Can you work these out from the model? Positions are in its coordinate system, mm. Coordinates: 2 decimals unless noted, no trailing zeros. Write each loop counter-clockwise with the first axis right and the second up, starting at its lowest first coordinate (ties: lowest second). Pieces come first, ordered by that corner, then holes. Notation, with made-up numbers: (-6.5, -2.5) -> (48.5, -2.5) arc R24 ccw to (48.5, 26.5) -> close; hole circle Ø9 at (28, 56.5). An arc over 180 degrees is marked (long way). Use one line per item in the form item = value.
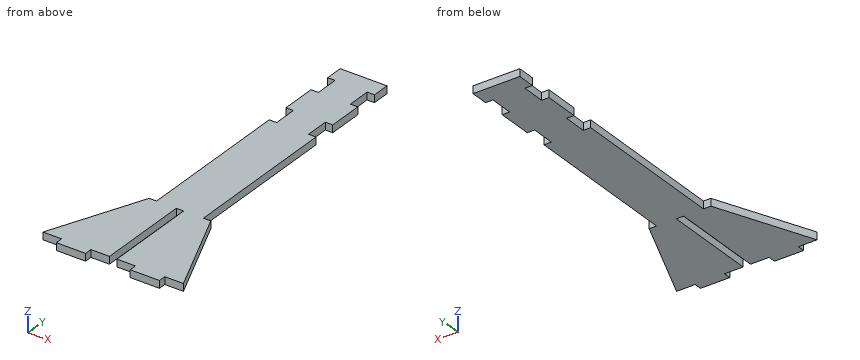
```python
from build123d import *

# Parameters (mm, degrees)
BOSS_EXTRU_1_DEPTH      = 6.35
ENL_V_MAT_EXTRU_1_REACH = 308.007
ESQUISSE2_W             = 6.35
ESQUISSE2_H             = 80
ENL_V_MAT_EXTRU_2_REACH = 308.007
ESQUISSE4_W             = 6.35
ESQUISSE4_H             = 20
SKETCH2_W               = 25
SKETCH2_H               = 6.35
BOSS_EXTRUDE2_DEPTH     = 6.35


with BuildPart() as part:
    # Esquisse1 → Boss.-Extru.1 (new body)
    with BuildSketch(Plane.XY):
        Polygon((-20, 300), (20, 300), (20, 80), (26.35, 80), (60, 0), (-60, 0), (-26.35, 80), (-20, 80), align=None)
    extrude(amount=BOSS_EXTRU_1_DEPTH)

    # Esquisse2 → Enlèv. mat.-Extru.1 (cut, up to next)
    with BuildSketch(Plane.XY.offset(6.35), mode=Mode.PRIVATE) as enl_v_mat_extru_1_sk1:
        with Locations((0, 40)):
            Rectangle(ESQUISSE2_W, ESQUISSE2_H)
    enl_v_mat_extru_1_tool1 = extrude(enl_v_mat_extru_1_sk1.sketch, amount=-ENL_V_MAT_EXTRU_1_REACH, mode=Mode.PRIVATE) & part.part
    add(enl_v_mat_extru_1_tool1.solids().sort_by_distance((0, 40, 6.35))[0], mode=Mode.SUBTRACT)

    # Esquisse4 → Enlèv. mat.-Extru.2 (cut, up to next)
    with BuildSketch(Plane.XY.offset(6.35), mode=Mode.PRIVATE) as enl_v_mat_extru_2_sk1:
        with Locations((16.825, 225)):
            Rectangle(ESQUISSE4_W, ESQUISSE4_H)
    enl_v_mat_extru_2_tool1 = extrude(enl_v_mat_extru_2_sk1.sketch, amount=-ENL_V_MAT_EXTRU_2_REACH, mode=Mode.PRIVATE) & part.part
    # Esquisse4 → Enlèv. mat.-Extru.2 (cut, up to next)
    with BuildSketch(Plane.XY.offset(6.35), mode=Mode.PRIVATE) as enl_v_mat_extru_2_sk2:
        with Locations((-16.825, 225)):
            Rectangle(ESQUISSE4_W, ESQUISSE4_H)
    enl_v_mat_extru_2_tool2 = extrude(enl_v_mat_extru_2_sk2.sketch, amount=-ENL_V_MAT_EXTRU_2_REACH, mode=Mode.PRIVATE) & part.part
    # Esquisse4 → Enlèv. mat.-Extru.2 (cut, up to next)
    with BuildSketch(Plane.XY.offset(6.35), mode=Mode.PRIVATE) as enl_v_mat_extru_2_sk3:
        with Locations((-16.825, 275)):
            Rectangle(ESQUISSE4_W, ESQUISSE4_H)
    enl_v_mat_extru_2_tool3 = extrude(enl_v_mat_extru_2_sk3.sketch, amount=-ENL_V_MAT_EXTRU_2_REACH, mode=Mode.PRIVATE) & part.part
    # Esquisse4 → Enlèv. mat.-Extru.2 (cut, up to next)
    with BuildSketch(Plane.XY.offset(6.35), mode=Mode.PRIVATE) as enl_v_mat_extru_2_sk4:
        with Locations((16.825, 275)):
            Rectangle(ESQUISSE4_W, ESQUISSE4_H)
    enl_v_mat_extru_2_tool4 = extrude(enl_v_mat_extru_2_sk4.sketch, amount=-ENL_V_MAT_EXTRU_2_REACH, mode=Mode.PRIVATE) & part.part
    add(enl_v_mat_extru_2_tool1.solids().sort_by_distance((16.825, 225, 6.35))[0], mode=Mode.SUBTRACT)
    add(enl_v_mat_extru_2_tool2.solids().sort_by_distance((-16.825, 225, 6.35))[0], mode=Mode.SUBTRACT)
    add(enl_v_mat_extru_2_tool3.solids().sort_by_distance((-16.825, 275, 6.35))[0], mode=Mode.SUBTRACT)
    add(enl_v_mat_extru_2_tool4.solids().sort_by_distance((16.825, 275, 6.35))[0], mode=Mode.SUBTRACT)

    # Sketch2 → Boss-Extrude2 (add)
    with BuildSketch(Plane(origin=(0, 0, 0), x_dir=(-1, 0, 0), z_dir=(0, -1, 0))):
        with Locations((31.5875, -3.175)):
            Rectangle(SKETCH2_W, SKETCH2_H)
        with Locations((-31.5875, -3.175)):
            Rectangle(SKETCH2_W, SKETCH2_H)
    extrude(amount=BOSS_EXTRUDE2_DEPTH)


solid = part.part
```
Q1. Suppose I cut it at B-B (y = 117.5). Write out the boundary of the cut face in (x, z).
Return value:
outline = (-20, 0) -> (20, 0) -> (20, 6.35) -> (-20, 6.35) -> close
Q2. Suppose I cut it at C-C (x = 7). Write out the boundary of the cut face in (y, z), then the cut area to 4 significant figures.
Return value:
outline = (0, 0) -> (300, 0) -> (300, 6.35) -> (0, 6.35) -> close
area = 1,905 mm2
Q3. Suppose I cut it at A-A (y = 23). Write out the boundary of the cut face in (x, z) (3 decimals).
Return value:
outline = (-50.326, 0) -> (-3.175, 0) -> (-3.175, 6.35) -> (-50.326, 6.35) -> close; (3.175, 0) -> (50.326, 0) -> (50.326, 6.35) -> (3.175, 6.35) -> close
Q4. If I drill on line 1 (Y direction, x = -16.5, z = 5); line 2 (X direction, y = 177, z = 4.25); line 3 (Y direction, x = -23.5, z = 1), over which ranges is the centre line in solid material (lowest first)? Write a range as from..to.
Return value:
line_1 = 0..215, 235..265, 285..300
line_2 = -20..20
line_3 = -6.35..80
Q5. Will these pins go through, and if not, where does the flat tip stop? pin 1 (1.9 mm diameter, centred on x = -16.5, z = 3, fed in from -Y); pin 2 (3 mm diameter, centred on y = -2.5, z = 4, fed in from -X); pin 3 (3 mm diameter, centred on y = 173.5, z = 1.5, fed in from +X).
Return value:
pin_1 = 0
pin_2 = -44.09
pin_3 = 20
